Check sheet for the modelled part. Datum: model origin and axes. Units: mm. A direction names the side the tool comes from. Give positions to 0.01 mm unless a question says otherwise; leave off trailing zeros. Loops run counter-clockwise (first coordinate to the right, second up) from the corner with the lowest first, then second, coordinate; pieces in that order, holes last.
```python
from build123d import *

# Parameters (mm, degrees)
SKETCH1_R      = 2
EXTRUDE1_DEPTH = 3
EXTRUDE3_DEPTH = 1.82
SKETCH2_R      = 1.475
EXTRUDE2_DEPTH = 16


with BuildPart() as part:
    # Sketch1 → Extrude1 (new body)
    with BuildSketch(Plane.XY):
        Circle(SKETCH1_R)
    extrude(amount=EXTRUDE1_DEPTH)

    # Sketch3 → Extrude3 (cut)
    with BuildSketch(Plane(origin=(0, 0, 0), x_dir=(-1, 0, 0), z_dir=(0, 0, -1))):
        Polygon((-1.443375673, 0), (-0.721687836, -1.25), (0.721687836, -1.25), (1.443375673, 0), (0.721687836, 1.25), (-0.721687836, 1.25), align=None)
    extrude(amount=-EXTRUDE3_DEPTH, mode=Mode.SUBTRACT)

    # Sketch2 → Extrude2 (add)
    with BuildSketch(Plane.XY.offset(3)):
        Circle(SKETCH2_R)
    extrude(amount=EXTRUDE2_DEPTH)


solid = part.part
```
(1) Release check for a two-part mould opening along X. For faces 3 (the face through (0, 0, 19)), 4 (the face through (1.08, 0.63, 0.9)), 5 (the face through (-1.474, 0.065, 10.888)) record: pulls with the +X half, pulls with the -X half, needs draft (parallel to the pull), parting line crosses it, or undercut.
(2) Gauge pin test, flat end, axial feed: pin 1 Ø0.8 at (x, y) = (0.5, -0.5) entering from -Z. Record the tip position at first contact, or that the pin passes through.
(3) Section check C-C on y = -0.3. Record the boundary of the cut face in (x, z).
(4) Section check A-A on x = 0. Record the boundary of the cut face in (y, z) (3 decimals).
(5) Access from +Z, -Z, +X, -X, +Y, -Y to the whole of each face (thin tool, end or side, straight path). Record for faces 1 (the face through (0, -2, 1)), 2 (the face through (-1.088, 0.616, 0.897)).
(6) Section check B-B on z = 1.5. Record the boundary of the cut face in (x, y), plus the area to 3 significant figures.
(7) Material ranges on line 1 (Z direction, x = -1.4, y = 0.7); line 2 (Z direction, x = 0.5, y = 0); line 3 (Y direction, x = 0.05, z = 13.75), recorded low to high.
(8) Section check D-D on z = 17.75. Record the boundary of the cut face in (x, y) (3 decimals).
Computed values:
1. face 3: needs draft
1. face 4: undercut
1. face 5: parting line crosses it
2. pin 1: stops at z = 1.82
3. outline: (-1.98, 0) - (-1.27, 0) - (-1.27, 1.82) - (1.27, 1.82) - (1.27, 0) - (1.98, 0) - (1.98, 3) - (1.44, 3) - (1.44, 19) - (-1.44, 19) - (-1.44, 3) - (-1.98, 3) - close
4. outline: (-2, 0) - (-1.25, 0) - (-1.25, 1.82) - (1.25, 1.82) - (1.25, 0) - (2, 0) - (2, 3) - (1.475, 3) - (1.475, 19) - (-1.475, 19) - (-1.475, 3) - (-2, 3) - close
5. face 1: +Z, -Z
5. face 2: -Z
6. outline: circle Ø4 at (0, 0); hole (-1.44, 0) - (-0.72, -1.25) - (0.72, -1.25) - (1.44, 0) - (0.72, 1.25) - (-0.72, 1.25) - close
6. area: 7.15 mm2
7. line 1: z = 0 to 3
7. line 2: z = 1.82 to 19
7. line 3: y = -1.47 to 1.47
8. outline: circle Ø2.95 at (0, 0)
